Part model, mm, in its own coordinate system. Round coordinates to 2 decimals unless told otherwise and drop trailing zeros. Write each loop counter-clockwise with the first axis right and the second up, starting at its lowest first coordinate (ties: lowest second). Pieces come first, ordered by that corner, then holes.
1) Saw through at B-B on z = -26.5. Write the cut outline in (x, y), and give its area (3 significant figures).
2) Flat gauge pins, fed straight in: pin 1 (1 mm diameter, centred on x = 1, z = 60, fed in from +Y); pin 2 (1.5 mm diameter, centred on x = 1.5, z = 21, fed in from -Y); pin 3 (0.9 mm diameter, centred on x = 1.5, z = -27.5, fed in from +Y). Where does each tip first touch, or does it go through?
3) Saw through at C-C on x = 2.15. Count the separate pieces of the cut face and the enclosed holes in it, and give its area (3 significant figures).
4) Drill centre lines: L1, parallel to Z at x = 0.25, y = -1.5; L2, parallel to Z at x = 0.2, y = 5.5; L3, parallel to Z at x = 1.25, y = 42.5. Where is each one in solid material? Low to high.
5) Saw through at A-A on y = -4.5. Write the cut outline in (x, z).
6) Saw through at D-D on z = 6. Write the cut outline in (x, y).
```python
from build123d import *

# Parameters (mm, degrees)
F0_R     = 3.175
F1_DEPTH = 3.048


with BuildPart() as f1:
    # F0 (on Right) → F1 (new body)
    with BuildSketch(Plane.YZ):
        with BuildLine():
            ThreePointArc((0, 72.1900944854), (6.7351920908, 74.9799023946), (9.525, 81.7150944854))
            ThreePointArc((9.525, 81.7150944854), (9.5063048942, 82.3115777274), (9.4502929642, 82.9057194854))
            ThreePointArc((9.4502929642, 82.9057194854), (0, 91.2400944854), (-9.4502929642, 82.9057194854))
            ThreePointArc((-9.4502929642, 82.9057194854), (-7.14375, 75.4148991759), (0, 72.1900944854))
        make_face()
        with BuildLine():
            ThreePointArc((3.175, 81.7150944854), (2.2450640303, 79.4700304552), (0, 78.5400944854))
            ThreePointArc((0, 78.5400944854), (-2.2450640303, 83.9601585157), (3.175, 81.7150944854))
        make_face(mode=Mode.SUBTRACT)
        with BuildLine():
            ThreePointArc((9.4502929642, 82.9057194854), (9.5063048942, 82.3115777274), (9.525, 81.7150944854))
            ThreePointArc((9.525, 81.7150944854), (6.7351920908, 74.9799023946), (0, 72.1900944854))
            Line((0, 72.1900944854), (0, 46.7900944854))
            Line((0, 46.7900944854), (0, 34.0900944854))
            ThreePointArc((0, 34.0900944854), (2.2450640303, 33.1601585157), (3.175, 30.9150944854))
            ThreePointArc((3.175, 30.9150944854), (2.2450640303, 28.6700304552), (0, 27.7400944854))
            Line((0, 27.7400944854), (0, 15.0400944854))
            ThreePointArc((0, 15.0400944854), (9.2843476683, 18.0381183895), (15.0619619516, 25.899825084))
            Line((15.0619619516, 25.899825084), (15.7504882737, 32.8994694854))
            Line((15.7504882737, 32.8994694854), (9.4502929642, 82.9057194854))
        make_face()
        with BuildLine():
            Line((0, 46.7900944854), (0, 72.1900944854))
            ThreePointArc((0, 72.1900944854), (-7.14375, 75.4148991759), (-9.4502929642, 82.9057194854))
            Line((-9.4502929642, 82.9057194854), (-15.7504882737, 32.8994694854))
            ThreePointArc((-15.7504882737, 32.8994694854), (-10.5003255158, 42.8213444854), (0, 46.7900944854))
        make_face()
        with Locations((-5.1205755983, 67.0795790052)):
            Circle(F0_R, mode=Mode.SUBTRACT)
        with BuildLine():
            ThreePointArc((15.0619619516, 25.899825084), (15.7987508259, 29.3610361396), (15.7504882737, 32.8994694854))
            Line((15.7504882737, 32.8994694854), (15.0619619516, 25.899825084))
        make_face()
        with BuildLine():
            Line((0, 34.0900944854), (0, 46.7900944854))
            ThreePointArc((0, 46.7900944854), (-10.5003255158, 42.8213444854), (-15.7504882737, 32.8994694854))
            Line((-15.7504882737, 32.8994694854), (-15.0619619516, 25.899825084))
            ThreePointArc((-15.0619619516, 25.899825084), (-9.2843476683, 18.0381183895), (0, 15.0400944854))
            Line((0, 15.0400944854), (0, 27.7400944854))
            ThreePointArc((0, 27.7400944854), (-3.175, 30.9150944854), (0, 34.0900944854))
        make_face()
        with BuildLine():
            Line((-15.0619619516, 25.899825084), (-15.7504882737, 32.8994694854))
            ThreePointArc((-15.7504882737, 32.8994694854), (-15.7987508259, 29.3610361396), (-15.0619619516, 25.899825084))
        make_face()
        with BuildLine():
            Line((10.1907467619, -23.6215556334), (15.0619619516, 25.899825084))
            ThreePointArc((15.0619619516, 25.899825084), (9.2843476683, 18.0381183895), (0, 15.0400944854))
            Line((0, 15.0400944854), (0, -23.3164066483))
            Line((0, -23.3164066483), (0.2772849675, -23.3247095949))
            Line((0.2772849675, -23.3247095949), (10.1907467619, -23.6215556334))
        make_face()
        with BuildLine():
            ThreePointArc((0, 15.0400944854), (-9.2843476683, 18.0381183895), (-15.0619619516, 25.899825084))
            Line((-15.0619619516, 25.899825084), (-9.2198489049, -33.4918242511))
            ThreePointArc((-9.2198489049, -33.4918242511), (-6.8640412592, -26.3629240764), (0, -23.3205590496))
            Line((0, -23.3205590496), (0, -23.3164066483))
            Line((0, -23.3164066483), (0, 15.0400944854))
        make_face()
        with BuildLine():
            Line((44.45, -24.6474055146), (10.1907467619, -23.6215556334))
            Line((10.1907467619, -23.6215556334), (9.3090587828, -32.5849055146))
            Line((9.3090587828, -32.5849055146), (36.5125, -32.5849055146))
            ThreePointArc((36.5125, -32.5849055146), (38.8373399243, -26.9722454389), (44.45, -24.6474055146))
        make_face()
        with BuildLine():
            Line((9.3090587828, -32.5849055146), (10.1907467619, -23.6215556334))
            Line((10.1907467619, -23.6215556334), (0.2772849675, -23.3247095949))
            ThreePointArc((0.2772849675, -23.3247095949), (6.6481944704, -26.1328030892), (9.264346465, -32.5849055146))
            Line((9.264346465, -32.5849055146), (9.3090587828, -32.5849055146))
        make_face()
        with BuildLine():
            ThreePointArc((0, -23.3205590496), (-6.8640412592, -26.3629240764), (-9.2198489049, -33.4918242511))
            ThreePointArc((-9.2198489049, -33.4918242511), (-6.2219814381, -39.4489467737), (0, -41.8492519796))
            Line((0, -41.8492519796), (0.5511328595, -41.8328440954))
            ThreePointArc((0.5511328595, -41.8328440954), (6.742922259, -38.937945325), (9.264346465, -32.5849055146))
            Line((9.264346465, -32.5849055146), (3.175, -32.5849055146))
            ThreePointArc((3.175, -32.5849055146), (-2.2450640303, -34.8299695448), (0, -29.4099055146))
            Line((0, -29.4099055146), (0, -23.3205590496))
        make_face()
        with BuildLine():
            Line((36.5125, -32.5849055146), (9.3090587828, -32.5849055146))
            Line((9.3090587828, -32.5849055146), (9.264346465, -32.5849055146))
            ThreePointArc((9.264346465, -32.5849055146), (6.742922259, -38.937945325), (0.5511328595, -41.8328440954))
            Line((0.5511328595, -41.8328440954), (44.6862042117, -40.5188902524))
            ThreePointArc((44.6862042117, -40.5188902524), (38.9214814227, -38.2804641869), (36.5125, -32.5849055146))
        make_face()
        with BuildLine():
            ThreePointArc((52.3875, -32.5849055146), (50.0626600757, -26.9722454389), (44.45, -24.6474055146))
            ThreePointArc((44.45, -24.6474055146), (38.8373399243, -26.9722454389), (36.5125, -32.5849055146))
            ThreePointArc((36.5125, -32.5849055146), (38.9214814227, -38.2804641869), (44.6862042117, -40.5188902524))
            ThreePointArc((44.6862042117, -40.5188902524), (50.1455586723, -38.1134240919), (52.3875, -32.5849055146))
        make_face()
        with BuildLine():
            ThreePointArc((47.625, -32.5849055146), (44.45, -35.7599055146), (41.275, -32.5849055146))
            ThreePointArc((41.275, -32.5849055146), (44.45, -29.4099055146), (47.625, -32.5849055146))
        make_face(mode=Mode.SUBTRACT)
        with BuildLine():
            Line((0.5511328595, -41.8328440954), (0, -41.8492519796))
            ThreePointArc((0, -41.8492519796), (0.2756885233, -41.8451491), (0.5511328595, -41.8328440954))
        make_face()
    extrude(amount=F1_DEPTH)


solid = f1.part
```
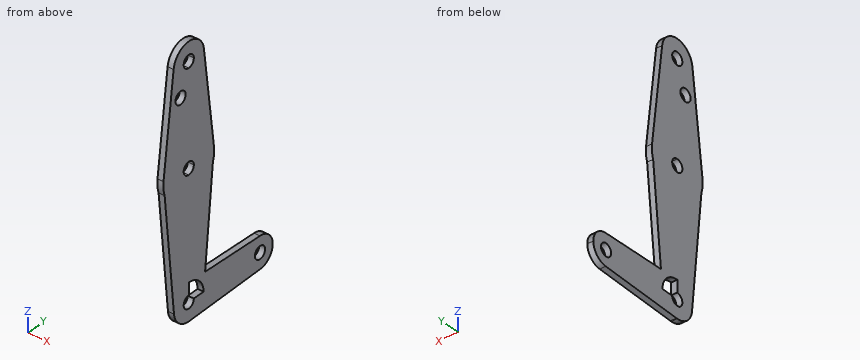
Completed:
1. outline: (0, -9.91) - (3.05, -9.91) - (3.05, 0) - (0, 0) - close; (0, 6.99) - (3.05, 6.99) - (3.05, 49.55) - (0, 49.55) - close
1. area: 160 mm2
2. pin 1: stops at y = 12.4
2. pin 2: stops at y = -14.65
2. pin 3: stops at y = 50.89
3. separate pieces: 1
3. enclosed holes: 5
3. area: 3,650 mm2
4. L1: z = -41.73 to -35.38, -29.79 to 28.12, 33.71 to 78.92, 84.51 to 91.12
4. L2: z = -41.69 to -32.58, -25.13 to 89.49
4. L3: z = -40.58 to -35.09, -30.08 to -24.59
5. outline: (0, -40.68) - (3.05, -40.68) - (3.05, 63.97) - (0, 63.97) - close; (0, 70.19) - (3.05, 70.19) - (3.05, 90.11) - (0, 90.11) - close
6. outline: (0, -13.1) - (3.05, -13.1) - (3.05, 13.1) - (0, 13.1) - close
